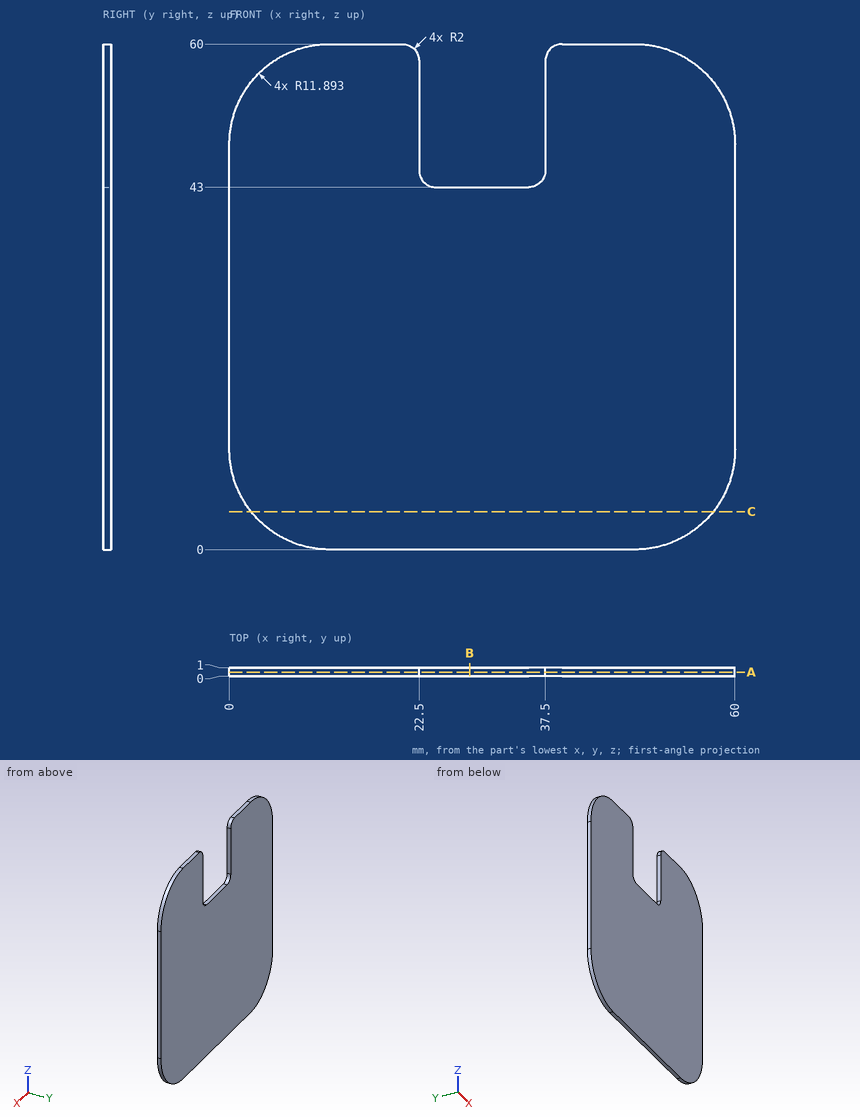
Here's the drawing with two shaded views (mm, measured from the low corner). I have some questions. Give positions to 0.01 mm unless a question says otherwise; leave off trailing zeros. Write each loop counter-clockwise with the first axis right and the second up, starting at its lowest first coordinate (ties: lowest second). Pieces come first, ordered by that corner, then holes. Notation, with made-up numbers: (68.25, 28.25) - (79.25, 28.25) arc R22 cw to (79.25, 35.25) - close; hole circle Ø2 at (34, 24.25). An arc over 180 degrees is marked (long way). One line per item, written item: value. Start each with the question number.
Item 1: I'm going to push a flat-ended pin straight in: pin 1 (0.5 mm diameter, centred on x = 31, y = 0.5, fed in from +Z). Where does the tip first touch, or does it pass through?
Item 2: Imagine slicing it at A-A, the plane y = 0.45. List the corners of the cut face in (x, z) for me, and give its area (3 significant figures).
Item 3: Imagine slicing it at C-C, the plane z = 4.5. List the corners of the cut face in (x, y) for me.
Item 4: Please list where these lines run through material, in increasing order: line 1 (X direction, y = 0.45, z = 55); line 2 (Z direction, x = 34.5, y = 0.55); line 3 (X direction, y = 0.45, z = 3.5) (1 decimal). Write a range as from..to.
Item 5: Imagine slicing it at B-B, the plane x = 28.5. List the corners of the cut face in (y, z) for me.
Geometry says:
1. pin 1: z = 43
2. outline: (0, 11.89) arc R11.89 ccw to (11.89, 0) - (48.11, 0) arc R11.89 ccw to (60, 11.89) - (60, 48.11) arc R11.89 ccw to (48.11, 60) - (39.5, 60) arc R2 ccw to (37.5, 58) - (37.5, 45) arc R2 cw to (35.5, 43) - (24.5, 43) arc R2 cw to (22.5, 45) - (22.5, 58) arc R2 ccw to (20.5, 60) - (11.89, 60) arc R11.89 ccw to (0, 48.11) - close
2. area: 3,220 mm^2
3. outline: (2.58, 0) - (57.42, 0) - (57.42, 1) - (2.58, 1) - close
4. line 1: 2.2..22.5, 37.5..57.8
4. line 2: 0..43
4. line 3: 3.5..56.5
5. outline: (0, 0) - (1, 0) - (1, 43) - (0, 43) - close
